Geometry check sheet. Reference: the model listing, model coordinates, mm. Coordinates: 2 decimals unless noted, no trailing zeros. Write each loop counter-clockwise with the first axis right and the second up, starting at its lowest first coordinate (ties: lowest second). Pieces come first, ordered by that corner, then holes. Notation, with made-up numbers: M 37,-0.75 L 76,-0.75 A10 cw 76,17.25 Z; hole C 45.25,62 d6. An arc over 180 degrees is marked long. Write each question's results on one line, items separated by ' | '.
```python
from build123d import *


with BuildPart() as part:
    # Esquisse1 → Révolution3 (revolve)
    with BuildSketch(Plane.XY, mode=Mode.PRIVATE) as r_volution3_sk:
        with BuildLine():
            Line((-0.625, 0), (-0.625, 132.922166212))
            Line((-0.625, 132.922166212), (0, 132.922166212))
            Line((0, 132.922166212), (0, 135))
            ThreePointArc((0, 135), (-1.698212195, 134.296577477), (-2.401634718, 132.598365282))
            Line((-2.401634718, 132.598365282), (-2.401634718, 127.386887788))
            ThreePointArc((-2.401634718, 127.386887788), (-2.174513205, 124.78141827), (-1.5, 122.254545197))
            Line((-1.5, 122.254545197), (-1.5, 0))
            Line((-1.5, 0), (-0.625, 0))
        make_face()
    revolve(r_volution3_sk.sketch.rotate(Axis((0, -0.0531705, 0), (0, 1, 0)), 270), axis=Axis((0, -0.0531705, 0), (0, 1, 0)))


solid = part.part
```
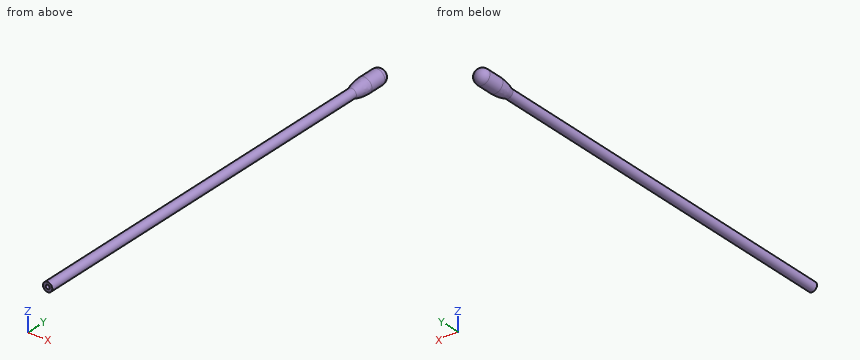
Q1. Scan lines: probe 1 along Z at (x, y) = (0.1, 72.5); probe 2 along X at (y, z) = (73, 0) (3 decimals); probe 3 along X at (y, z) = (36.5, -0.45). Record each from-to range of solid material in increasing order.
Geometry check:
probe 1: z = -1.5 to -0.62, 0.62 to 1.5 | probe 2: x = -1.5 to -0.625, 0.625 to 1.5 | probe 3: x = -1.43 to -0.43, 0.43 to 1.43
Q2. Depth check by flat-ended pin: P1, Ø0.8, axis at x = 0, z = 0, coming from the -Y side. Enter the tip coordinate at first touch or a pass-through.
Geometry check:
P1: stops at y = 132.92
Q3. Sectioned sample at A-A on y = 76. Record the cut outline in (x, z) (3 decimals).
Geometry check:
outline: C 0,0 d3; hole C 0,0 d1.25
